from build123d import *

# Parameters (mm, degrees)
F1_DEPTH = 31.75
F3_DEPTH = 25.4
F5_DEPTH = 12.7
F7_DEPTH = 12.7


with BuildPart() as f1:
    # F0 (on Top) → F1 (new body)
    with BuildSketch(Plane.XY):
        Polygon((0, 38.1), (0, 0), (31.75, 0), (31.75, 12.7), (69.85, 12.7), (69.85, 25.4), (31.395252, 25.4), (31.395252, 38.1), align=None)
    extrude(amount=F1_DEPTH)

    # F2 (on face) → F3 (cut)
    with BuildSketch(Plane.XZ.offset(-12.7)):
        Polygon((69.85, 31.75), (57.15, 31.75), (69.85, 0), align=None)
    extrude(amount=-F3_DEPTH, mode=Mode.SUBTRACT)

    # F4 (on face) → F5 (cut)
    with BuildSketch(Plane.XZ):
        Polygon((31.75, 31.75), (19.05, 31.75), (31.75, 0), align=None)
    extrude(amount=-F5_DEPTH, mode=Mode.SUBTRACT)

    # F6 (on face) → F7 (cut)
    with BuildSketch(Plane(origin=(0, 38.1, 0), x_dir=(-1, 0, 0), z_dir=(0, 1, 0))):
        Polygon((-31.395252, 0), (-19.556509, 31.75), (-31.395252, 31.75), align=None)
    extrude(amount=-F7_DEPTH, mode=Mode.SUBTRACT)


solid = f1.part
Work out the finished part from the listing and answer in its coordinate system (mm). A direction names the side the tool comes from. Give positions to 0.01 mm unless a question says otherwise; leave off trailing zeros. Loops run counter-clockwise (first coordinate to the right, second up) from the corner with the lowest first, then second, coordinate; pieces in that order, holes last. Notation, with made-up numbers: (66, -17.75) - (107, -17.75) arc R20 ccw to (107, -8.75) - close; hole circle Ø9 at (67.25, 7). An arc over 180 degrees is marked (long way). Answer in a Markdown table with one row per item. Add a question column.
Q1. The part is cut by section A-A (x = 24). Determine the outline of the cut face in (y, z) (3 decimals), and give its area (3 significant figures).
Q2. A tool of negligible diameter and unlimited length cuts with its end or side. For faces 1 (the flat face through (44, 12.7, 16)), 2 (the flat face through (25.56, 31.84, 15.65)), 3 (the flat face through (12, 38.1, 16)), from which of +Z, -Z, +X, -X, +Y, -Y can it reach the whole face along a straight path? Write none if from no direction.
Q3. The part is cut by section D-D (x = 44). Determine the outline of the cut face in (y, z).
Q4. Consider line 1 along Y through (x, z) = (45, 7); line 2 along X through (y, z) = (31.5, 25.5); line 3 along X through (y, z) = (36, 10). Determine where each line is inside the solid, lowest interval first.
Q5. The part is cut by section B-B (z = 2). Determine the outline of the cut face in (x, y).
Q6. The part is cut by section C-C (y = 18). Determine the outline of the cut face in (x, z), and give its area (3 significant figures).
Q7. Each of these flat-tipped pins is pushed along its axis until it touches: P1, Ø1, axis at x = 60.5, z = 10, coming from the +Y side; P2, Ø1.5, axis at x = 42, z = 8.5, coming from the -Y side. Where does it stop, or does it pass through?
Solution:
| question | item | result |
|---|---|---|
| 1 | outline | (0, 0) - (38.1, 0) - (38.1, 19.833) - (25.4, 19.833) - (25.4, 31.75) - (12.7, 31.75) - (12.7, 19.375) - (0, 19.375) - close |
| 1 | area | 901 mm² |
| 2 | face 1 | +Z, +X, -Y |
| 2 | face 2 | +Z, +X, +Y |
| 2 | face 3 | +Z, -Z, +X, -X, +Y |
| 3 | outline | (12.7, 0) - (25.4, 0) - (25.4, 31.75) - (12.7, 31.75) - close |
| 4 | line 1 | y = 12.7 to 25.4 |
| 4 | line 2 | x = 0 to 21.89 |
| 4 | line 3 | x = 0 to 27.67 |
| 5 | outline | (0, 0) - (30.95, 0) - (30.95, 12.7) - (69.05, 12.7) - (69.05, 25.4) - (30.65, 25.4) - (30.65, 38.1) - (0, 38.1) - close |
| 6 | outline | (0, 0) - (69.85, 0) - (57.15, 31.75) - (0, 31.75) - close |
| 6 | area | 2,020 mm² |
| 7 | P1 | stops at y = 25.4 |
| 7 | P2 | stops at y = 12.7 |
